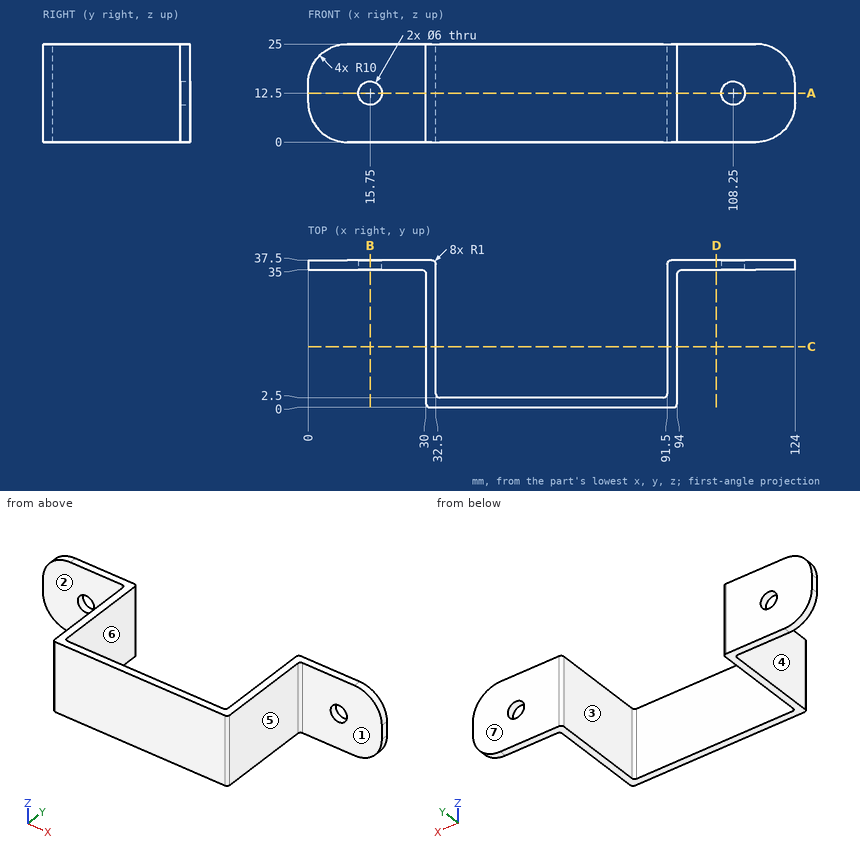
Geometry check sheet. Reference: drawing and pictorial views, mm from the part's lowest x, y, z. A direction names the side the tool comes from. Give positions to 0.01 mm unless a question says otherwise; leave off trailing zeros. Order: outer loops, then holes, each group sorted by start corner. A loop starts at its lowest first (then second) coordinate and runs counter-clockwise, first axis right, second up. Notation, with made-up numbers: M 41.25,30 L 86.25,30 A26 cw 86.25,45 Z; hole C 43,75.5 d5. An arc over 180 degrees is marked long. Answer in a Markdown table with one row per item.
1) Cross-section at D-D, the plane x = 104. Enter the section's corners in (y, z), plus the area to 3 significant figures.
Filled sheet:
| item | result |
|---|---|
| outline | M 35,0 L 37.5,0 L 37.5,25 L 35,25 Z |
| area | 62.5 mm2 |
2) Cross-section at A-A, the plane z = 12.5. Enter the section's corners in (x, y).
Filled sheet:
| item | result |
|---|---|
| outline | M 0,35 L 12.75,35 L 12.75,37.5 L 0,37.5 Z; M 18.75,35 L 29,35 A1 cw 30,34 L 30,1 A1 ccw 31,0 L 93,0 A1 ccw 94,1 L 94,34 A1 cw 95,35 L 105.25,35 L 105.25,37.5 L 92.5,37.5 A1 ccw 91.5,36.5 L 91.5,3.5 A1 cw 90.5,2.5 L 33.5,2.5 A1 cw 32.5,3.5 L 32.5,36.5 A1 ccw 31.5,37.5 L 18.75,37.5 Z; M 111.25,35 L 124,35 L 124,37.5 L 111.25,37.5 Z |
3) Gauge pin test, flat ends, axial feed: P1, Ø5, axis at x = 15.75, z = 12.5, coming from the +Y side; P2, Ø1, axis at x = 34.5, z = 13, coming from the +Y side; P3, Ø8, axis at y = 19.5, z = 9.5, coming from the +X side; P4, Ø7.5, axis at x = 9.5, z = 12, coming from the -Y side. Record the tip position at first contact, or that the pin passes through.
Filled sheet:
| item | result |
|---|---|
| P1 | passes through |
| P2 | stops at y = 2.5 |
| P3 | stops at x = 94 |
| P4 | stops at y = 35 |
4) Cross-section at C-C, the plane y = 15.5. Enter the section's corners in (x, z).
Filled sheet:
| item | result |
|---|---|
| outline | M 30,0 L 32.5,0 L 32.5,25 L 30,25 Z; M 91.5,0 L 94,0 L 94,25 L 91.5,25 Z |
5) Cross-section at B-B, the plane x = 15.75. Enter the section's corners in (y, z), plus the area to 3 significant figures.
Filled sheet:
| item | result |
|---|---|
| outline | M 35,0 L 37.5,0 L 37.5,9.5 L 35,9.5 Z; M 35,15.5 L 37.5,15.5 L 37.5,25 L 35,25 Z |
| area | 47.5 mm2 |
6) Thickness scan on L1, parallel to X at y = 29, z = 6; L2, parallel to Z at x = 15.75, y = 35.95; L3, parallel to Y at x = 6, z = 18.5. Record the ranges inside material, lowest first. Write a range as [from, to].
Filled sheet:
| item | result |
|---|---|
| L1 | x = [30, 32.5], [91.5, 94] |
| L2 | z = [0, 9.5], [15.5, 25] |
| L3 | y = [35, 37.5] |
7) Access from +Z, -Z, +X, -X, +Y, -Y to the whole of each face (thin tool, end or side, straight path). Record for the marked faces 1, 2 and 3.
Filled sheet:
| item | result |
|---|---|
| face 1 | +Z, -Z, +X, -Y |
| face 2 | +Z, -Z, -X, -Y |
| face 3 | +Z, -Z, +Y |
8) Release check for a two-part mould opening along X. For the marked faces 4, 5, 6 and 7 record: +X half, -X half, draft (parallel to the pull), parting line (faces both ways), or undercut.
Filled sheet:
| item | result |
|---|---|
| face 4 | -X half |
| face 5 | +X half |
| face 6 | undercut |
| face 7 | draft |
